from build123d import *

# Parameters (mm, degrees)
SKETCH_1_R          = 10.125
EXTRUDE_1_DEPTH     = 3.5
SKETCH_2_R          = 12
EXTRUDE_2_DEPTH     = 2
CUT_EXTRUDE_1_DEPTH = 21.223748416
SKETCH_4_R          = 1.5
CUT_EXTRUDE_2_DEPTH = 18.839562775


with BuildPart() as part:
    # 草图1 → 凸台-拉伸1 (new, symmetric)
    with BuildSketch(Plane.XY):
        Circle(SKETCH_1_R)
    extrude(amount=EXTRUDE_1_DEPTH, both=True)

    # 草图2 → 凸台-拉伸2 (add)
    with BuildSketch(Plane.XY.offset(3.5)):
        Circle(SKETCH_2_R)
    extrude_2 = extrude(amount=EXTRUDE_2_DEPTH)

    # 镜向1: 凸台-拉伸2 across plane
    add(extrude_2.mirror(Plane.XY))

    # 草图3 → 切除-拉伸1 (cut, through all)
    with BuildSketch(Plane.XY.offset(5.5)):
        with BuildLine():
            Line((-2, 2.236067977), (-2, -2.236067977))
            ThreePointArc((-2, -2.236067977), (3, 0), (-2, 2.236067977))
        make_face()
    extrude(amount=-CUT_EXTRUDE_1_DEPTH, mode=Mode.SUBTRACT)

    # 草图4 → 切除-拉伸2 (cut, through all)
    with BuildSketch(Plane(origin=(0, 0, 0), x_dir=(1, 0, 0), z_dir=(0, 1, 0))):
        with Locations(Location((0, 0, 0), (0, 0, 270))):
            Circle(SKETCH_4_R)
    extrude(amount=-CUT_EXTRUDE_2_DEPTH, mode=Mode.SUBTRACT)


solid = part.part
Model file for the job. Use its own axes, mm. A direction names the side the tool comes from. Coordinates: 2 decimals unless noted, no trailing zeros. Loops run counter-clockwise (first coordinate to the right, second up) from the corner with the lowest first, then second, coordinate; pieces in that order, holes last. Notation, with made-up numbers: (-7, 83) -> (-3, 83) arc R13 ccw to (-3, 100) -> close; hole circle Ø8 at (54.5, -3). An arc over 180 degrees is marked (long way). Use one line per item in the form item = value. Start each with the question number.
(1) Cut at D-D on z = -4. Give the cut face in (x, y).
(2) Cut at C-C on y = -5.5. Give the cut face in (x, z), and give its area (3 significant figures).
(3) Tool access for faces 1 (the flat face through (-3, 0, 5.5)), 2 (the cylindrical face through (-1.33, -6.31, 0.69)), 3 (the cylindrical face through (5.44, 8.54, 0.05)): list every direction of +Z, -Z, +X, -X, +Y, -Y with a clear straight run to the whole face (end or side of a thin tool).
(4) Cut at A-A on x = 0. Give the cut face in (y, z) (3 decimals), and give its area (3 significant figures).
(5) Flat gauge pins, fed straight in: pin 1 (5 mm diameter, centred on y = -7.5, z = -4, fed in from +X); pin 2 (1.5 mm diameter, centred on y = 1, z = -1, fed in from +X); pin 3 (1.5 mm diameter, centred on x = 2.5, z = 0.5, fed in from -Y). Where does each tip first touch, or does it go through?
(6) Probe probe 1 along Y at (x, z) = (0, 3) (3 decimals); probe 2 along Z at (x, y) = (8.75, 7.75); probe 3 along Z at (x, y) = (0, -6.5). List the from-to ranges inside material, lowest first. Write a range as from..to.
(7) Pull direction Y, two halves, no side cores. Call faces 4 (the flat face through (-5, -9, 3.5)), 5 (the flat face through (-2, 0, 0)), 6 (the cylindrical face through (-11.99, 0.53, -4.49)): pulls with the +Y half, pulls with the -Y half, needs draft (parallel to the pull), parting line crosses it, or undercut.
(8) Cut at B-B on y = 0. Give the cut face in (x, z) (3 decimals), and give its area (3 significant figures).
Values:
q1.outline = circle Ø24 at (0, 0); hole (-2, -2.24) arc R3 ccw (long way) to (-2, 2.24) -> close
q2.outline = (-10.67, -5.5) -> (10.67, -5.5) -> (10.67, -3.5) -> (8.5, -3.5) -> (8.5, 3.5) -> (10.67, 3.5) -> (10.67, 5.5) -> (-10.67, 5.5) -> (-10.67, 3.5) -> (-8.5, 3.5) -> (-8.5, -3.5) -> (-10.67, -3.5) -> close; hole circle Ø3 at (0, 0)
q2.area = 197 mm2
q3.face_1 = +Z, +X, -X, +Y, -Y
q3.face_2 = -Y
q3.face_3 = none
q4.outline = (-12, -5.5) -> (-3, -5.5) -> (-3, -1.5) -> (-10.125, -1.5) -> (-10.125, -3.5) -> (-12, -3.5) -> close; (-12, 3.5) -> (-10.125, 3.5) -> (-10.125, 1.5) -> (-3, 1.5) -> (-3, 5.5) -> (-12, 5.5) -> close; (3, -5.5) -> (12, -5.5) -> (12, -3.5) -> (10.125, -3.5) -> (10.125, 3.5) -> (12, 3.5) -> (12, 5.5) -> (3, 5.5) -> close
q4.area = 150 mm2
q5.pin_1 = 10.91
q5.pin_2 = 10.12
q5.pin_3 = -9.97
q6.probe_1 = -10.125..-3, 3..10.125
q6.probe_2 = -5.5..-3.5, 3.5..5.5
q6.probe_3 = -5.5..-1.5, 1.5..5.5
q7.face_4 = needs draft
q7.face_5 = undercut
q7.face_6 = parting line crosses it
q8.outline = (-12, -5.5) -> (-2, -5.5) -> (-2, 5.5) -> (-12, 5.5) -> (-12, 3.5) -> (-10.125, 3.5) -> (-10.125, -3.5) -> (-12, -3.5) -> close; (3, -5.5) -> (12, -5.5) -> (12, -3.5) -> (10.125, -3.5) -> (10.125, 3.5) -> (12, 3.5) -> (12, 5.5) -> (3, 5.5) -> close
q8.area = 183 mm2
